The model under review builds one solid part; all positions refer to its coordinate system, in mm. Coordinates: 2 decimals unless noted, no trailing zeros. One line per item, written item: value. Start each with the question number.
1. We need section A-A, the plane z = 2.25. Count the separate pieces of the cut face and the enclosed holes in it, then the cut area to 3 significant figures.
2. Insertion check: P1, Ø9, axis at x = 292.1, y = -138.11, coming from the -Z side; P2, Ø2, axis at y = 98, z = 4, coming from the -X side. Each pin has a flat end and moves straight along its axis. Give the tip position at first contact, or say it passes through.
3. To check wall thickness, follow line 1 (Y direction, x = 584.2, z = 5); line 2 (Y direction, x = 292.1, z = 5.5); line 3 (Y direction, x = 357.5, z = 9.25). State the ranges of each line that lie inside material, in increasing order.
from build123d import *

# Parameters (mm, degrees)
F0_R     = 3.81
F1_DEPTH = 12.7
F2_SIZE  = 5.08


with BuildPart() as f1:
    # F0 (on Top) → F1 (new body)
    with BuildSketch(Plane.XY):
        with BuildLine():
            Line((603.25, -157.1625), (603.25, 157.1625))
            Line((603.25, 157.1625), (-584.2, 157.1625))
            Line((-584.2, 157.1625), (-584.2, 141.9225))
            ThreePointArc((-584.2, 141.9225), (-581.505923, 140.806577), (-580.39, 138.1125))
            ThreePointArc((-580.39, 138.1125), (-584.2, 134.3025), (-588.01, 138.1125))
            Line((-588.01, 138.1125), (-603.25, 138.1125))
            Line((-603.25, 138.1125), (-603.25, -157.1625))
            Line((-603.25, -157.1625), (603.25, -157.1625))
        make_face()
        with Locations((-584.2, -138.1125)):
            Circle(F0_R, mode=Mode.SUBTRACT)
        with Locations((-292.1, -138.1125)):
            Circle(F0_R, mode=Mode.SUBTRACT)
        with Locations((0, -138.1125)):
            Circle(F0_R, mode=Mode.SUBTRACT)
        with Locations((292.1, -138.1125)):
            Circle(F0_R, mode=Mode.SUBTRACT)
        with Locations((584.2, -138.1125)):
            Circle(F0_R, mode=Mode.SUBTRACT)
        with Locations((-584.2, 0)):
            Circle(F0_R, mode=Mode.SUBTRACT)
        with Locations((-292.1, 0)):
            Circle(F0_R, mode=Mode.SUBTRACT)
        with Locations((-292.1, 138.1125)):
            Circle(F0_R, mode=Mode.SUBTRACT)
        Circle(F0_R, mode=Mode.SUBTRACT)
        with Locations((292.1, 0)):
            Circle(F0_R, mode=Mode.SUBTRACT)
        with Locations((584.2, 0)):
            Circle(F0_R, mode=Mode.SUBTRACT)
        with Locations((0, 138.1125)):
            Circle(F0_R, mode=Mode.SUBTRACT)
        with Locations((292.1, 138.1125)):
            Circle(F0_R, mode=Mode.SUBTRACT)
        with Locations((584.2, 138.1125)):
            Circle(F0_R, mode=Mode.SUBTRACT)
        with BuildLine():
            Line((-584.2, 141.9225), (-584.2, 157.1625))
            Line((-584.2, 157.1625), (-603.25, 157.1625))
            Line((-603.25, 157.1625), (-603.25, 138.1125))
            Line((-603.25, 138.1125), (-588.01, 138.1125))
            ThreePointArc((-588.01, 138.1125), (-586.894077, 140.806577), (-584.2, 141.9225))
        make_face()
    extrude(amount=F1_DEPTH)

    # F2
    f2_edges = [f1.edges().sort_by_distance(p)[0] for p in [
        (0, 157.1625, 0),
        (603.25, 0, 0),
        (0, -157.1625, 0),
        (-603.25, 0, 0),
        (0, -157.1625, 12.7),
        (603.25, 0, 12.7),
        (0, 157.1625, 12.7),
        (-603.25, 0, 12.7),
    ]]
    chamfer(f2_edges, length=F2_SIZE)


solid = f1.part
Findings below:
1. separate pieces: 1
1. enclosed holes: 15
1. area: 370,000 mm2
2. P1: z = 0
2. P2: x = -603.17
3. line 1: -157.08 to -141.92, -134.3 to -3.81, 3.81 to 134.3, 141.92 to 157.08
3. line 2: -157.16 to -141.92, -134.3 to -3.81, 3.81 to 134.3, 141.92 to 157.16
3. line 3: -155.53 to 155.53
